Part model, mm, in its own coordinate system. Face numbers are marked on the shaded views. Coordinates: 2 decimals unless noted, no trailing zeros. Loops run counter-clockwise (first coordinate to the right, second up) from the corner with the lowest first, then second, coordinate; pieces in that order, holes last. Notation, with made-up numbers: (4.25, 68.25) - (43.25, 68.25) arc R14 ccw to (43.25, 87.25) - close; hole circle Ø4 at (11, -36.5). An arc over 180 degrees is marked (long way). Use a Markdown table: item, result. Add a question column.
1. Band-saw the part on A-A, the plane x = 54. Give the cut face in (y, z) (3 decimals).
2. Pull direction Y, two halves, no side cores. Call the marked faces 1, 2, 3 and 4: pulls with the +Y half, pulls with the -Y half, needs draft (parallel to the pull), parting line crosses it, or undercut.
3. Drop flat-ended pins along their axis: pin 1 (5 mm diameter, centred on y = -21.5, z = -3, fed in from -X); pin 2 (1.5 mm diameter, centred on x = 53.5, y = -20.5, fed in from -Z); pin 3 (4 mm diameter, centred on y = -42, z = -6.5, fed in from +X); pin 4 (8 mm diameter, centred on y = -49, z = -7.5, fed in from +X). Give the stop position or say it passes through.
4. Wall check: probe 1 along Y at (x, z) = (54, -5.75); probe 2 along X at (y, z) = (-50.5, -12.5); probe 3 along X at (y, z) = (-42.5, -1). Give the ranges that are in metal, low to high. Write a range as [from, to].
5. Band-saw the part on C-C, the plane z = -9.75. Give the cut face in (x, y).
6. Band-saw the part on B-B, the plane y = -17.5. Give the cut face in (x, z).
7. Band-saw the part on D-D, the plane x = 51. Count the separate pieces of the cut face and the enclosed holes in it, plus the area to 3 significant figures.
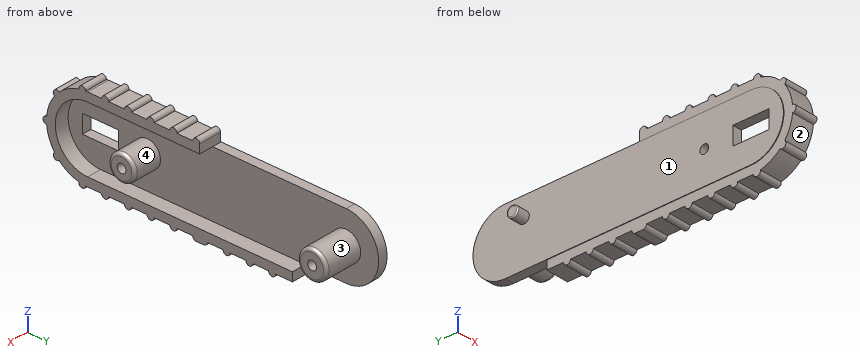
from build123d import *

# Parameters (mm, degrees)
PAD122_DEPTH                      = 1.6
PAD123_DEPTH                      = 4.05
POCKET098_DEPTH                   = 0.1
SKETCH216_R                       = 0.75
SKETCH216_W                       = 6
SKETCH216_H                       = 3
POCKET099_DEPTH                   = 1.6
PAD124_DEPTH                      = 3.95
SKETCH218_R                       = 2.25
PAD125_DEPTH                      = 4.9
SKETCH219_R                       = 0.75
POCKET100_DEPTH                   = 4.9
SKETCH220_R                       = 2.475
PAD126_DEPTH                      = 6.5
SKETCH221_R                       = 0.75
POCKET101_DEPTH                   = 6.5
FILLET044_R                       = 0.5
SKETCH222_R                       = 0.95
PAD127_DEPTH                      = 2.2
FILLET045_R                       = 0.2
SKETCH356_W                       = 6.2
SKETCH356_H                       = 3.1
POCKET172_DEPTH                   = 5
BODY018_ROLL_ANGLE                = -90
BODY018_PITCH_ANGLE               = 0.040452
BODY018_PLACEMENT_ANGLE           = 90
PART_MIRRORING002_PLACEMENT_ANGLE = 180


with BuildPart() as right_inner_leg001:
    # Sketch214 → Pad122 (new body)
    with BuildSketch(Plane.XY):
        with BuildLine():
            Line((0, 5.55), (42.05, 5.55))
            ThreePointArc((42.049962, -5.55), (47.599981, -1.9e-05), (42.05, 5.55))
            Line((42.049962, -5.55), (0, -5.55))
            ThreePointArc((0, 5.55), (-5.55, 0), (0, -5.55))
        make_face()
    extrude(amount=PAD122_DEPTH)

    # Sketch215 (on Face5 of Pad122) → Pad123 (join)
    with BuildSketch(Plane(origin=(0, 0, 0), x_dir=(1, 0, 0), z_dir=(0, 0, -1))):
        with BuildLine():
            Line((19.17, 5.55), (0, 5.55))
            ThreePointArc((0, 5.55), (-5.55, 0), (0, -5.55))
            Line((0, -5.55), (35.05, -5.55))
            Line((35.05, -5.55), (35.05, -7.05))
            Line((0, -7.05), (35.05, -7.05))
            ThreePointArc((0, 7.05), (-7.05, 0), (0, -7.05))
            Line((19.17, 7.05), (0, 7.05))
            Line((19.17, 5.55), (19.17, 7.05))
        make_face()
    extrude(amount=-PAD123_DEPTH)

    # Sketch215 (on Face5 of Pad122) → Pocket098 (cut)
    with BuildSketch(Plane(origin=(0, 0, 0), x_dir=(1, 0, 0), z_dir=(0, 0, -1))):
        with BuildLine():
            Line((19.17, 5.55), (0, 5.55))
            ThreePointArc((0, 5.55), (-5.55, 0), (0, -5.55))
            Line((0, -5.55), (35.05, -5.55))
            Line((35.05, -5.55), (35.05, -7.05))
            Line((0, -7.05), (35.05, -7.05))
            ThreePointArc((0, 7.05), (-7.05, 0), (0, -7.05))
            Line((19.17, 7.05), (0, 7.05))
            Line((19.17, 5.55), (19.17, 7.05))
        make_face()
    extrude(amount=-POCKET098_DEPTH, mode=Mode.SUBTRACT)

    # Sketch216 (on Face1 of Pocket098) → Pocket099 (cut)
    with BuildSketch(Plane(origin=(0, 0, 0), x_dir=(1, 0, 0), z_dir=(0, 0, -1))):
        with Locations((8, 0)):
            Circle(SKETCH216_R)
        Rectangle(SKETCH216_W, SKETCH216_H)
    extrude(amount=-POCKET099_DEPTH, mode=Mode.SUBTRACT)

    # Sketch217 (on Face11 of Pocket099) → Pad124 (join)
    with BuildSketch(Plane(origin=(0, 0, 0.1), x_dir=(1, 0, 0), z_dir=(0, 0, -1))):
        with BuildLine():
            ThreePointArc((19.17, 7.05), (18.57, 7.65), (17.97, 7.05))
            Line((19.17, 7.05), (17.97, 7.05))
        make_face()
        with BuildLine():
            ThreePointArc((15.27, 7.05), (14.67, 7.65), (14.07, 7.05))
            Line((15.27, 7.05), (14.07, 7.05))
        make_face()
        with BuildLine():
            ThreePointArc((11.37, 7.05), (10.77, 7.65), (10.17, 7.05))
            Line((11.37, 7.05), (10.17, 7.05))
        make_face()
        with BuildLine():
            ThreePointArc((7.47, 7.05), (6.87, 7.65), (6.27, 7.05))
            Line((7.47, 7.05), (6.27, 7.05))
        make_face()
        with BuildLine():
            ThreePointArc((3.57, 7.05), (2.97, 7.65), (2.37, 7.05))
            Line((3.57, 7.05), (2.37, 7.05))
        make_face()
        with BuildLine():
            ThreePointArc((-0.33, 7.042272), (-1.006549, 7.583492), (-1.51849, 6.884525))
            Line((-0.33, 7.042272), (-1.51849, 6.884525))
        make_face()
        with BuildLine():
            ThreePointArc((-4.890151, 5.078279), (-5.755669, 5.039323), (-5.679917, 4.176247))
            Line((-4.890151, 5.078279), (-5.679917, 4.176247))
        make_face()
        with BuildLine():
            ThreePointArc((-7.024468, 0.599457), (-7.65, 0), (-7.024468, -0.599457))
            Line((-7.024468, 0.599457), (-7.024468, -0.599457))
        make_face()
        with BuildLine():
            ThreePointArc((-5.677552, -4.179462), (-5.733191, -5.026164), (-4.886489, -5.081803))
            Line((-4.886489, -5.081803), (-5.677552, -4.179462))
        make_face()
        with BuildLine():
            ThreePointArc((-1.513526, -6.885618), (-1.001082, -7.584216), (-0.324923, -7.042508))
            Line((-0.324923, -7.042508), (-1.513526, -6.885618))
        make_face()
        with BuildLine():
            ThreePointArc((2.375077, -7.05), (2.975077, -7.65), (3.575077, -7.05))
            Line((3.575077, -7.05), (2.375077, -7.05))
        make_face()
        with BuildLine():
            ThreePointArc((6.275077, -7.05), (6.875077, -7.65), (7.475077, -7.05))
            Line((7.475077, -7.05), (6.275077, -7.05))
        make_face()
        with BuildLine():
            ThreePointArc((10.175077, -7.05), (10.775077, -7.65), (11.375077, -7.05))
            Line((11.375077, -7.05), (10.175077, -7.05))
        make_face()
        with BuildLine():
            ThreePointArc((14.075077, -7.05), (14.675077, -7.65), (15.275077, -7.05))
            Line((15.275077, -7.05), (14.075077, -7.05))
        make_face()
        with BuildLine():
            ThreePointArc((23.175077, -7.05), (23.775077, -7.65), (24.375077, -7.05))
            Line((24.375077, -7.05), (23.175077, -7.05))
        make_face()
        with BuildLine():
            ThreePointArc((27.075077, -7.05), (27.675077, -7.65), (28.275077, -7.05))
            Line((28.275077, -7.05), (27.075077, -7.05))
        make_face()
        with BuildLine():
            ThreePointArc((30.975077, -7.05), (31.575077, -7.65), (32.175077, -7.05))
            Line((32.175077, -7.05), (30.975077, -7.05))
        make_face()
        with BuildLine():
            ThreePointArc((17.975077, -7.05), (18.150813, -7.474264), (18.575077, -7.65))
            Line((19.875077, -7.65), (18.575077, -7.65))
            ThreePointArc((19.875077, -7.65), (20.299341, -7.474264), (20.475077, -7.05))
            Line((20.475077, -7.05), (17.975077, -7.05))
        make_face()
    extrude(amount=-PAD124_DEPTH)

    # Sketch218 (on Face12 of Pad124) → Pad125 (join)
    with BuildSketch(Plane.XY.offset(1.6)):
        with Locations((8, 0)):
            Circle(SKETCH218_R)
    extrude(amount=PAD125_DEPTH)

    # Sketch219 (on Face61 of Pad125) → Pocket100 (cut)
    with BuildSketch(Plane.XY.offset(6.5)):
        with Locations((8, 0)):
            Circle(SKETCH219_R)
    extrude(amount=-POCKET100_DEPTH, mode=Mode.SUBTRACT)

    # Sketch220 (on Face12 of Pocket100) → Pad126 (join)
    with BuildSketch(Plane.XY.offset(1.6)):
        with Locations((42.049981, 0)):
            Circle(SKETCH220_R)
    extrude(amount=PAD126_DEPTH)

    # Sketch221 (on Face62 of Pad126) → Pocket101 (cut)
    with BuildSketch(Plane.XY.offset(8.1)):
        with Locations((42.049981, 0)):
            Circle(SKETCH221_R)
    extrude(amount=-POCKET101_DEPTH, mode=Mode.SUBTRACT)

    # Fillet044
    fillet044_edges = [right_inner_leg001.edges().sort_by_distance(p)[0] for p in [
        (39.574981, 0, 8.1),
        (5.75, 0, 6.5),
    ]]
    fillet(fillet044_edges, radius=FILLET044_R)

    # Sketch222 (on Face5 of Fillet044) → Pad127 (join)
    with BuildSketch(Plane(origin=(0, 0, 0), x_dir=(1, 0, 0), z_dir=(0, 0, -1))):
        with Locations((38.899981, 2.2)):
            Circle(SKETCH222_R)
    extrude(amount=PAD127_DEPTH)

    # Fillet045
    fillet045_edges = [right_inner_leg001.edges().sort_by_distance(p)[0] for p in [
        (37.949981, -2.2, -2.2),
    ]]
    fillet(fillet045_edges, radius=FILLET045_R)

    # Sketch356 (on Face16 of Fillet045) → Pocket172 (cut)
    with BuildSketch(Plane.XY.offset(1.6)):
        Rectangle(SKETCH356_W, SKETCH356_H)
    extrude(amount=-POCKET172_DEPTH, mode=Mode.SUBTRACT)


with BuildPart() as right_inner_leg001_1:
    # Body018 roll: moved
    add(right_inner_leg001.part.rotate(Axis((0, 0, 0), (1, 0, 0)), BODY018_ROLL_ANGLE))


with BuildPart() as right_inner_leg001_2:
    # Body018 pitch: moved
    add(right_inner_leg001_1.part.rotate(Axis((0, 0, 0), (0, 1, 0)), BODY018_PITCH_ANGLE))


with BuildPart() as right_inner_leg001_3:
    # Body018 placement: moved
    add(right_inner_leg001_2.part.moved(Location((-10.89, -44.504589, -8.889998))).rotate(Axis((-10.89, -44.504589, -8.889998), (0, 0, 1)), BODY018_PLACEMENT_ANGLE))


with BuildPart() as left_inner_leg:
    # Part__Mirroring002: instance of Right_Inner_Leg001
    add(right_inner_leg001_3.part.mirror(Plane(origin=(0, 0, 0), x_dir=(0, 1, 0), z_dir=(0, 0, 1))))


with BuildPart() as left_inner_leg_1:
    # Part__Mirroring002 placement: moved
    add(left_inner_leg.part.moved(Location((37.71, -6.5, 2.5))).rotate(Axis((37.71, -6.5, 2.5), (0, -1, 0)), PART_MIRRORING002_PLACEMENT_ANGLE))


solid = left_inner_leg_1.part
Geometry check:
| question | item | result |
|---|---|---|
| 1 | outline | circle Ø4.5 at (-43.005, -6.396); circle Ø4.95 at (-8.955, -6.42); hole circle Ø1.5 at (-43.005, -6.396); hole circle Ø1.5 at (-8.955, -6.42) |
| 2 | face 1 | needs draft |
| 2 | face 2 | pulls with the -Y half |
| 2 | face 3 | undercut |
| 2 | face 4 | undercut |
| 3 | pin 1 | stops at x = 48.6 |
| 3 | pin 2 | passes through |
| 3 | pin 3 | stops at x = 55.1 |
| 3 | pin 4 | stops at x = 54.96 |
| 4 | probe 1 | y = [-45.16, -43.39], [-42.62, -40.85], [-11.34, -9.29], [-8.62, -6.57] |
| 4 | probe 2 | x = [48.7, 52.65] |
| 4 | probe 3 | x = [48.6, 50.2] |
| 5 | outline | (48.6, -55.42) - (48.7, -55.42) - (48.7, -57.2) - (52.65, -57.2) - (52.65, -55.42) - (50.2, -55.42) - (50.2, -4.51) - (48.6, -4.51) - close |
| 6 | outline | (48.6, -11.96) - (48.7, -11.96) - (48.7, -13.46) - (52.65, -13.46) - (52.65, -11.96) - (50.2, -11.96) - (50.2, -0.86) - (48.6, -0.86) - close |
| 7 | separate pieces | 3 |
| 7 | enclosed holes | 2 |
| 7 | area | 154 mm^2 |
